Verification items for this drawing (mm, ordinates from the low corner). A direction names the side the tool comes from. Coordinates: 2 decimals unless noted, no trailing zeros. Order: outer loops, then holes, each group sorted by start corner. A loop starts at its lowest first (then second) coordinate and runs counter-clockwise, first axis right, second up. Notation, with made-up numbers: M 40.25,-19.75 L 44.25,-19.75 A23 cw 44.25,12.25 Z; hole C -25.5,69 d11. An arc over 180 degrees is marked long. Answer as a JSON object with one key per item and string values. Group by question number.
(1) Access from +Z, -Z, +X, -X, +Y, -Y to the whole of each face (thin tool, end or side, straight path). Record for the marked faces 1 and 2.
(2) Cross-section at D-D (y = 34). Enter the section's corners in (x, z), plus the area to 3 significant figures.
(3) Gauge pin test, flat ends, axial feed: pin 1 Ø3.5 at (x, y) = (5.5, 6) entering from +Z; pin 2 Ø0.9 at (x, y) = (5.5, 36) entering from +Z; pin 3 Ø6 at (x, y) = (16, 24.5) entering from +Z. Record the tip position at first contact, or that the pin passes through.
(4) Cross-section at A-A (y = 21.15). Enter the section's corners in (x, z).
(5) Material ranges on line 1 (Y direction, x = 36.65, z = 38.6); line 2 (X direction, y = 6.5, z = 36); line 3 (Z direction, x = 22, y = 4.5), recorded low to high.
(6) Cross-section at C-C (z = 55.5). Enter the section's corners in (x, y), plus the area to 3 significant figures.
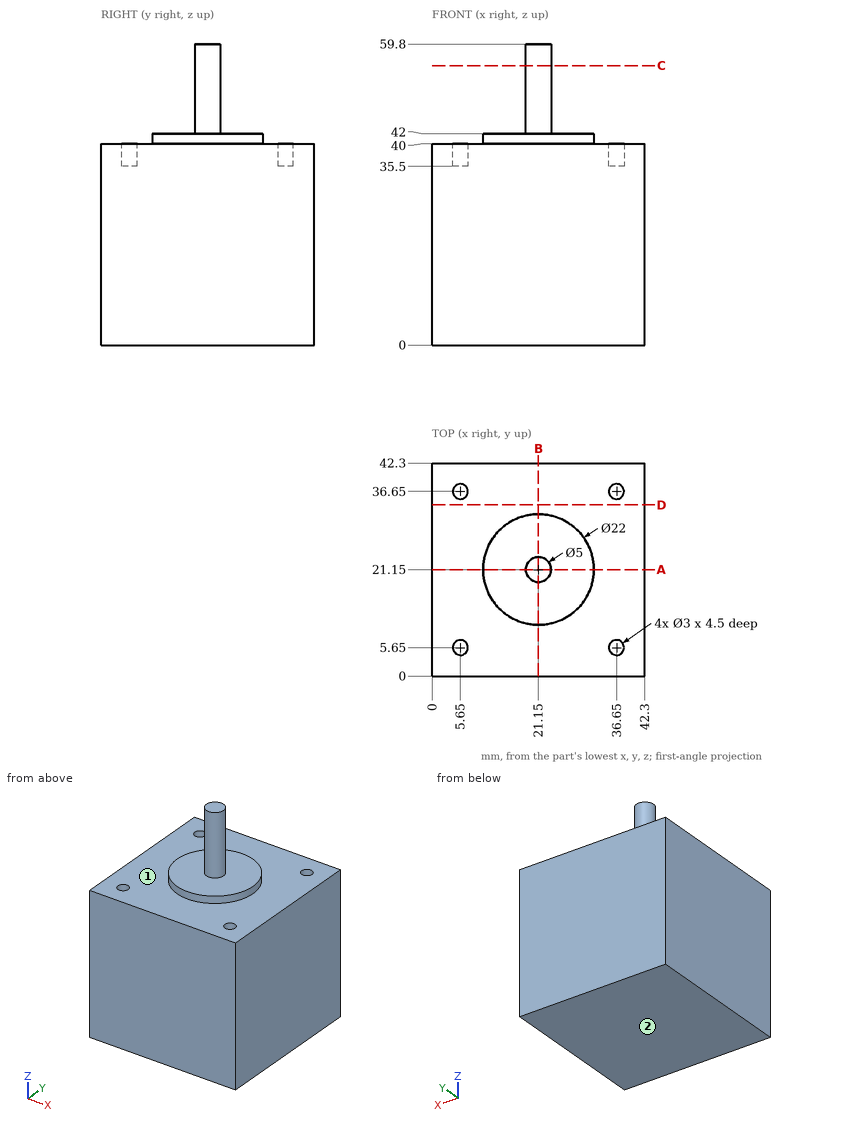
Taken from the geometry:
{
 "1": {"face 1": "+Z", "face 2": "-Z, +X, -X, +Y, -Y"},
 "2": {"outline": "M 0,0 L 42.3,0 L 42.3,40 L 0,40 Z", "area": "1,690 mm²"},
 "3": {"pin 1": "stops at z = 40", "pin 2": "stops at z = 35.5", "pin 3": "stops at z = 42"},
 "4": {"outline": "M 0,0 L 42.3,0 L 42.3,40 L 32.15,40 L 32.15,42 L 23.65,42 L 23.65,59.8 L 18.65,59.8 L 18.65,42 L 10.15,42 L 10.15,40 L 0,40 Z"},
 "5": {"line 1": "y = 0 to 4.15, 7.15 to 35.15, 38.15 to 42.3", "line 2": "x = 0 to 4.41, 6.89 to 35.41, 37.89 to 42.3", "line 3": "z = 0 to 40"},
 "6": {"outline": "C 21.15,21.15 d5", "area": "19.6 mm²"}
}
